from build123d import *

# Parameters (mm, degrees)
F0_W     = 92.7
F0_H     = 92.7
F1_DEPTH = 6.35
F2_W     = 30
F2_H     = 20
F2_W_2   = 40
F2_H_2   = 40
F2_R     = 1.905
F3_DEPTH = 6.351


with BuildPart() as f1:
    # F0 (on Top) → F1 (new body)
    with BuildSketch(Plane.XY):
        Rectangle(F0_W, F0_H)
    extrude(amount=F1_DEPTH)

    # F2 (on face) → F3 (cut, through all)
    with BuildSketch(Plane.XY.offset(6.35)):
        with Locations((0, -28.35)):
            Rectangle(F2_W, F2_H)
        with Locations((0, 20)):
            Rectangle(F2_W_2, F2_H_2)
        with Locations((0, -4.445)):
            Circle(F2_R)
    extrude(amount=-F3_DEPTH, mode=Mode.SUBTRACT)


solid = f1.part
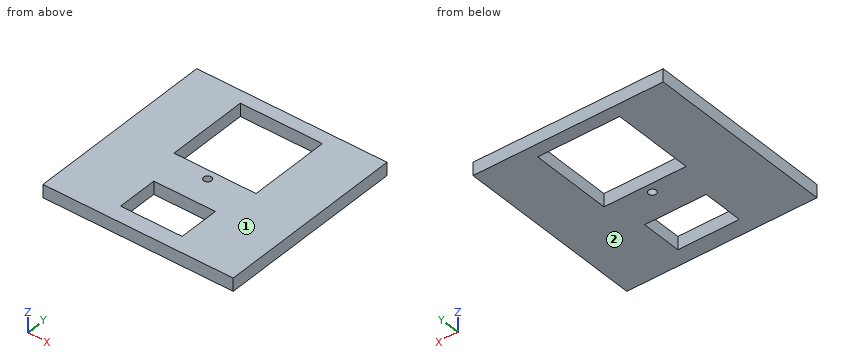
Verification items for the finished model (mm, model axes). Face numbers are marked on the shaded views. Coordinates: 2 decimals unless noted, no trailing zeros. Write each loop counter-clockwise with the first axis right and the second up, starting at its lowest first coordinate (ties: lowest second). Pieces come first, ordered by that corner, then holes. Notation, with made-up numbers: M 0,89 L 14,89 A22 ccw 14,107 Z; hole C 14,-7 d7. An arc over 180 degrees is marked long. Use CSV: the item, a comma, the result in double quotes.
Q1. Thickness scan on line 1 along Y through (x, z) = (-14.5, 3.25); line 2 along Y through (x, z) = (0, 1.75); line 3 along X through (y, z) = (-25.5, 1). Record the ranges inside material, lowest first. Write a range as [from, to].
Computed values:
line 1,"[-46.35, -38.35], [-18.35, 0], [40, 46.35]"
line 2,"[-46.35, -38.35], [-18.35, -6.35], [-2.54, 0], [40, 46.35]"
line 3,"[-46.35, -15], [15, 46.35]"
Q2. Mould release check, pull along Z, two halves, no side actions. Record for the marked faces 1 and 2: pulls with the +Z half, pulls with the -Z half, needs draft (parallel to the pull), parting line crosses it, or undercut.
Computed values:
face 1,"pulls with the +Z half"
face 2,"pulls with the -Z half"
Q3. Section check A-A, the plane y = 14. Enter the section's corners in (x, z), and give its area (3 significant figures).
Computed values:
outline,"M -46.35,0 L -20,0 L -20,6.35 L -46.35,6.35 Z; M 20,0 L 46.35,0 L 46.35,6.35 L 20,6.35 Z"
area,"335 mm²"
Q4. Section check C-C, the plane z = 2.5. Enter the section's corners in (x, y) (3 decimals).
Computed values:
outline,"M -46.35,-46.35 L 46.35,-46.35 L 46.35,46.35 L -46.35,46.35 Z; hole M -20,0 L 20,0 L 20,40 L -20,40 Z; hole M -15,-38.35 L 15,-38.35 L 15,-18.35 L -15,-18.35 Z; hole C 0,-4.445 d3.81"
Q5. Go/stop test with a flat-tipped pin: P1, Ø3, axis at x = 0, y = -4.445, coming from the -Z side. Record where the tip stops, or that it passes through.
Computed values:
P1,"through"
Q6. Section check B-B, the plane x = 0. Enter the section's corners in (y, z).
Computed values:
outline,"M -46.35,0 L -38.35,0 L -38.35,6.35 L -46.35,6.35 Z; M -18.35,0 L -6.35,0 L -6.35,6.35 L -18.35,6.35 Z; M -2.54,0 L 0,0 L 0,6.35 L -2.54,6.35 Z; M 40,0 L 46.35,0 L 46.35,6.35 L 40,6.35 Z"
